Source: CAD feature listing. Evaluate the final solid. Frame: model axes, mm. A direction names the side the tool comes from. Round coordinates to 2 decimals unless told otherwise and drop trailing zeros. Write each loop counter-clockwise with the first axis right and the second up, starting at its lowest first coordinate (ties: lowest second). Pieces come first, ordered by that corner, then holes.
from build123d import *

# Parameters (mm, degrees)
SKETCH1_R           = 1.7
BOSS_EXTRUDE1_DEPTH = 5


with BuildPart() as part:
    # Sketch1 → Boss-Extrude1 (new body)
    with BuildSketch(Plane(origin=(0, 0, 0), x_dir=(1, 0, 0), z_dir=(0, 1, 0))):
        Polygon((-30, 132.790561914), (30, 132.790561914), (130, -40.414518843), (100, -92.37604307), (-100, -92.37604307), (-130, -40.414518843), align=None)
        with Locations(Location((-27.5, 127.790561914, 0), (0, 0, 270))):
            Circle(SKETCH1_R, mode=Mode.SUBTRACT)
        with Locations(Location((-27.5, 72.790561914, 0), (0, 0, 270))):
            Circle(SKETCH1_R, mode=Mode.SUBTRACT)
        with Locations(Location((27.5, 127.790561914, 0), (0, 0, 90))):
            Circle(SKETCH1_R, mode=Mode.SUBTRACT)
        with Locations(Location((27.5, 72.790561914, 0), (0, 0, 90))):
            Circle(SKETCH1_R, mode=Mode.SUBTRACT)
        with Locations(Location((76.788475773, -12.579582353, 0), (0, 0, 270))):
            Circle(SKETCH1_R, mode=Mode.SUBTRACT)
        with Locations(Location((49.288475773, -60.210979561, 0), (0, 0, 90))):
            Circle(SKETCH1_R, mode=Mode.SUBTRACT)
        with Locations(Location((96.919872981, -87.710979561, 0), (0, 0, 90))):
            Circle(SKETCH1_R, mode=Mode.SUBTRACT)
        with Locations(Location((124.419872981, -40.079582353, 0), (0, 0, 270))):
            Circle(SKETCH1_R, mode=Mode.SUBTRACT)
        with Locations(Location((-49.288475773, -60.210979561, 0), (0, 0, 270))):
            Circle(SKETCH1_R, mode=Mode.SUBTRACT)
        with Locations(Location((-76.788475773, -12.579582353, 0), (0, 0, 90))):
            Circle(SKETCH1_R, mode=Mode.SUBTRACT)
        with Locations(Location((-124.419872981, -40.079582353, 0), (0, 0, 90))):
            Circle(SKETCH1_R, mode=Mode.SUBTRACT)
        with Locations(Location((-96.919872981, -87.710979561, 0), (0, 0, 270))):
            Circle(SKETCH1_R, mode=Mode.SUBTRACT)
        Polygon((-72.168783649, 0), (-36.084391824, -62.5), (36.084391824, -62.5), (72.168783649, 0), (36.084391824, 62.5), (-36.084391824, 62.5), align=None, mode=Mode.SUBTRACT)
    extrude(amount=BOSS_EXTRUDE1_DEPTH)


solid = part.part
1) Section query B-B on z = -5. Return the cut outline in (x, y).
Taken from the geometry:
outline: (-103.78, 0) - (-69.28, 0) - (-69.28, 5) - (-103.78, 5) - close; (69.28, 0) - (103.78, 0) - (103.78, 5) - (69.28, 5) - close
2) Reachability of faces 1 (the face through (-54.38, 2.46, 30.81)), 2 (the face through (-80.7, 2.465, -44.976)) from +Z, -Z, +X, -X, +Y, -Y: full face, straight path, thin tool, end or side. Return the list, or none.
Taken from the geometry:
face 1: +Y, -Y
face 2: -Z, -X, +Y, -Y
3) Section query D-D on x = 112. Return the cut outline in (y, z).
Taken from the geometry:
outline: (0, 9.24) - (5, 9.24) - (5, 71.59) - (0, 71.59) - close
4) Section query C-C on y = 4.2. State how many separate pieces and enclosed holes the cut face has, then the cut area to 3 significant figures.
Taken from the geometry:
separate pieces: 1
enclosed holes: 13
area: 26,000 mm2
5) Pull-direction query (X, two-part tool) for faces 3 (the face through (53.874, 2.465, 31.688)), 4 (the face through (115.21, 2.46, 66.03)), 5 (the face through (60, 5, -22)); classes: released by +X, released by -X, zero draft, split by the parting line, or undercut.
Taken from the geometry:
face 3: undercut
face 4: released by +X
face 5: zero draft
6) Contact query for flat-ended pins moving along their axis: P1, Ø1.5, axis at y = 0.5, z = -45.5, coming from the +X side; P2, Ø3, axis at y = 2, z = -34.5, coming from the -X side; P3, Ø5.5, axis at x = -27.5, z = -127.79, coming from the -Y side; P4, Ø3, axis at y = 3.5, z = 59, coming from the +X side. Output: stop coordinate, or through.
Taken from the geometry:
P1: stops at x = 80.83
P2: stops at x = -87.61
P3: stops at y = 0
P4: stops at x = 120.14
7) Section query A-A on x = 17.5. Return the cut outline in (y, z).
Taken from the geometry:
outline: (0, -132.79) - (5, -132.79) - (5, -62.5) - (0, -62.5) - close; (0, 62.5) - (5, 62.5) - (5, 92.38) - (0, 92.38) - close
8) Material intervals for line 1 (Z direction, x = -5, y = 4.2); line 2 (X direction, y = 2.15, z = -46); line 3 (X direction, y = 2.95, z = 51), sorted ascending.
Taken from the geometry:
line 1: z = -132.79 to -62.5, 62.5 to 92.38
line 2: x = -80.11 to -45.61, 45.61 to 80.11
line 3: x = -123.89 to -42.72, 42.72 to 123.89
